The listing builds one solid part. Answer for the finished solid, in the listing's coordinates (mm). Face numbers are marked on the shaded views. A direction names the side the tool comes from. Coordinates: 2 decimals unless noted, no trailing zeros. Loops run counter-clockwise (first coordinate to the right, second up) from the corner with the lowest first, then second, coordinate; pieces in that order, holes last. Notation, with made-up numbers: M 57,45.25 L 87,45.25 A20 cw 87,79.25 Z; hole C -30.5,79 d6. An arc over 180 degrees is marked long. Return JSON: item names as keys, results as strings. Group by question number.
1. Section C-C (z = -11) is taken. Write down the section's boundary in (x, y), then the cut area to 3 significant figures.
2. Which of the six approach directions +Z, -Z, +X, -X, +Y, -Y give full straight-line access (tool end or side, diameter ignored) to the marked faces 4 and 5?
3. The mould has two halves that part along X. Classify the marked faces 1, 2 and 3: pulls with the +X half, pulls with the -X half, needs draft (parallel to the pull), parting line crosses it, or undercut.
4. Given P1, Ø10, axis at x = -1.5, y = -10.5, coming from the -Z side; P2, Ø1.5, axis at x = 0, y = -1, coming from the -Z side; P3, Ø3, axis at y = -7, z = -16, coming from the +X side; P4, Ø6, axis at x = 1, z = -4, coming from the +Y side, each flat-ended and moving along its own axis, determine where each tip first touches the part or whether it passes through.
5. Section A-A (x = 0) is taken. Write down the section's boundary in (y, z).
6. Straight lines are drawn through the part: L1, parallel to Y at x = 0, z = -9.5; L2, parallel to Z at x = 2, y = -11; L3, parallel to Y at x = -2, z = -8.5. For each, find the intervals that lie inside material, in ascending order. Write a range as from..to.
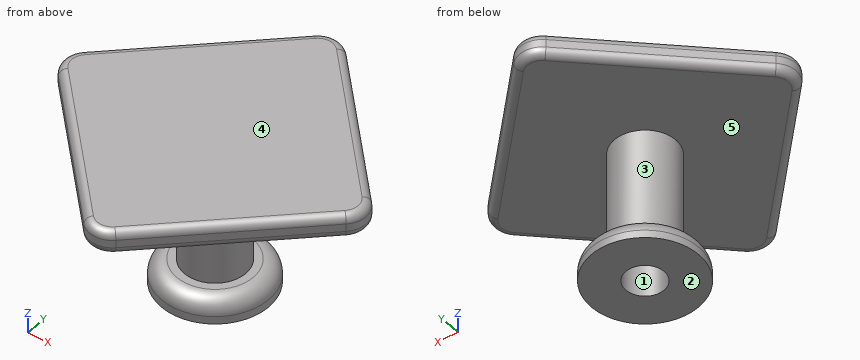
```python
from build123d import *

# Parameters (mm, degrees)
BOSS_EXTRUDE1_DEPTH = 1.5
FILLET1_R           = 3
FILLET3_R           = 1
BOSS_EXTRUDE2_START = -1.5
SKETCH1_3_R         = 4
SKETCH1_3_R_2       = 2.5
BOSS_EXTRUDE2_DEPTH = 17
BOSS_EXTRUDE3_START = -15.5
SKETCH1_4_R         = 7
SKETCH1_4_R_2       = 4
BOSS_EXTRUDE3_DEPTH = 3
FILLET4_R           = 2


with BuildPart() as part:
    # Sketch1 → Boss-Extrude1 (new, symmetric)
    with BuildSketch(Plane.XY):
        Polygon((-21.213203436, 0), (0, 21.213203436), (21.213203436, 0), (0, -21.213203436), align=None)
    extrude(amount=BOSS_EXTRUDE1_DEPTH, both=True)

    # Fillet1
    fillet1_edges = [part.edges().sort_by_distance(p)[0] for p in [
        (-21.213203436, 0, 0),
        (0, 21.213203436, 0),
        (21.213203436, 0, 0),
        (0, -21.213203436, 0),
    ]]
    fillet(fillet1_edges, radius=FILLET1_R)

    # Fillet3
    fillet3_edges = [part.edges().sort_by_distance(p)[0] for p in [
        (-10.606601718, -10.606601718, -1.5),
        (-10.606601718, -10.606601718, 1.5),
        (-10.606601718, 10.606601718, -1.5),
        (10.606601718, 10.606601718, -1.5),
        (10.606601718, -10.606601718, -1.5),
        (0, 19.970562748, -1.5),
        (0, -19.970562748, -1.5),
        (19.970562748, 0, -1.5),
        (-19.970562748, 0, -1.5),
        (-10.606601718, 10.606601718, 1.5),
        (10.606601718, -10.606601718, 1.5),
        (10.606601718, 10.606601718, 1.5),
        (0, 19.970562748, 1.5),
        (0, -19.970562748, 1.5),
        (19.970562748, 0, 1.5),
        (-19.970562748, 0, 1.5),
    ]]
    fillet(fillet3_edges, radius=FILLET3_R)

    # Sketch1<3> → Boss-Extrude2 (add)
    with BuildSketch(Plane.XY.offset(BOSS_EXTRUDE2_START)):
        Circle(SKETCH1_3_R)
        Circle(SKETCH1_3_R_2, mode=Mode.SUBTRACT)
    extrude(amount=-BOSS_EXTRUDE2_DEPTH)

    # Sketch1<4> → Boss-Extrude3 (add)
    with BuildSketch(Plane.XY.offset(BOSS_EXTRUDE3_START)):
        Circle(SKETCH1_4_R)
        Circle(SKETCH1_4_R_2, mode=Mode.SUBTRACT)
    extrude(amount=-BOSS_EXTRUDE3_DEPTH)

    # Fillet4
    fillet4_edges = [part.edges().sort_by_distance(p)[0] for p in [
        (-7, 0, -15.5),
    ]]
    fillet(fillet4_edges, radius=FILLET4_R)


solid = part.part
```
Worked out:
{
 "1": {"outline": "C 0,0 d8; hole C 0,0 d5", "area": "30.6 mm^2"},
 "2": {"face 4": "+Z, +X, -X, +Y, -Y", "face 5": "none"},
 "3": {"face 1": "undercut", "face 2": "needs draft", "face 3": "parting line crosses it"},
 "4": {"P1": "z = -18.5", "P2": "z = -1.5", "P3": "x = 3.81", "P4": "y = 19.77"},
 "5": {"outline": "M -19.97,-0.5 A1 ccw -18.97,-1.5 L -4,-1.5 L -4,-15.5 L -5,-15.5 A2 ccw -7,-17.5 L -7,-18.5 L -2.5,-18.5 L -2.5,-1.5 L 2.5,-1.5 L 2.5,-18.5 L 7,-18.5 L 7,-17.5 A2 ccw 5,-15.5 L 4,-15.5 L 4,-1.5 L 18.97,-1.5 A1 ccw 19.97,-0.5 L 19.97,0.5 A1 ccw 18.97,1.5 L -18.97,1.5 A1 ccw -19.97,0.5 Z"},
 "6": {"L1": "-4..-2.5, 2.5..4", "L2": "-1.5..1.5", "L3": "-3.46..-1.5, 1.5..3.46"}
}
